from build123d import *

# Parameters (mm, degrees)
SKETCH1_W           = 13
SKETCH1_H           = 12
BOSS_EXTRUDE1_DEPTH = 3
SKETCH2_W           = 13
SKETCH2_H           = 1.9
BOSS_EXTRUDE2_DEPTH = 3
CHAMFER1_SIZE       = 13
CHAMFER1_SIZE_2     = 2
CUT_EXTRUDE1_REACH  = 17.129
CUT_EXTRUDE1_START  = -0.5


with BuildPart() as part:
    # Sketch1 → Boss-Extrude1 (new body)
    with BuildSketch(Plane(origin=(0, 0, 0), x_dir=(1, 0, 0), z_dir=(0, 1, 0))):
        Rectangle(SKETCH1_W, SKETCH1_H)
    extrude(amount=BOSS_EXTRUDE1_DEPTH)

    # Sketch2 → Boss-Extrude2 (add)
    with BuildSketch(Plane.XZ):
        with Locations((0, 5.05)):
            Rectangle(SKETCH2_W, SKETCH2_H)
        with Locations((0, -5.05)):
            Rectangle(SKETCH2_W, SKETCH2_H)
    extrude(amount=BOSS_EXTRUDE2_DEPTH)

    # Chamfer1
    # the kernel refuses this chamfer: 13, 2 mm, written as the material it takes off along each edge
    with BuildSketch(Plane(origin=(6.5, -3, 39.785461495), x_dir=(-0.9999828835142526, -0.005850869894363576, 0), z_dir=(0, 0, -1))) as chamfer1_piece_1:
        Polygon((CHAMFER1_SIZE * 0.999982883514, CHAMFER1_SIZE * 0.00585086989436), (-CHAMFER1_SIZE_2 * 0.00585086989436, CHAMFER1_SIZE_2 * 0.999982883514), (0, 0), align=None)
    extrude(amount=69.470922991, mode=Mode.SUBTRACT)
    with BuildSketch(Plane(origin=(6.5, -3, -39.785461495), x_dir=(-0.9999828835142526, -0.005850869894363576, 0), z_dir=(0, 0, 1))) as chamfer1_piece_2:
        Polygon((CHAMFER1_SIZE * 0.999982883514, -CHAMFER1_SIZE * 0.00585086989436), (-CHAMFER1_SIZE_2 * 0.00585086989436, -CHAMFER1_SIZE_2 * 0.999982883514), (0, 0), align=None)
    extrude(amount=69.470922991, mode=Mode.SUBTRACT)
    with BuildSketch(Plane(origin=(6.5, 3, 39.785461495), x_dir=(0.23997968203750644, -0.9707779108576674, 0), z_dir=(0, 0, -1))) as chamfer1_piece_3:
        Polygon((CHAMFER1_SIZE_2 * 0.970777910858, CHAMFER1_SIZE_2 * 0.239979682038), (-CHAMFER1_SIZE * 0.239979682038, CHAMFER1_SIZE * 0.970777910858), (0, 0), align=None)
    extrude(amount=79.570922991, mode=Mode.SUBTRACT)

    # Sketch5 → Cut-Extrude1 (cut, up to next)
    with BuildSketch(Plane.ZY.offset(6.5).offset(CUT_EXTRUDE1_START), mode=Mode.PRIVATE) as cut_extrude1_sk1:
        with BuildLine():
            Line((-2, 3), (2, 3))
            ThreePointArc((2, 3), (0, 1), (-2, 3))
        make_face()
    cut_extrude1_tool1 = extrude(cut_extrude1_sk1.sketch, amount=-CUT_EXTRUDE1_REACH, mode=Mode.PRIVATE) & part.part
    add(cut_extrude1_tool1.solids().sort_by_distance((-6, 2.151174, 0))[0], mode=Mode.SUBTRACT)


solid = part.part
CAD build for the part. Positions are in the model's coordinates, mm. A direction names the side the tool comes from. Coordinates: 2 decimals unless noted, no trailing zeros. Loops run counter-clockwise (first coordinate to the right, second up) from the corner with the lowest first, then second, coordinate; pieces in that order, holes last. Notation, with made-up numbers: (66, 42) - (121, 42) arc R29 cw to (121, 79) - close; hole circle Ø4 at (4, -31). An arc over 180 degrees is marked (long way). Use one line per item in the form item = value. Start each with the question number.
1) Band-saw the part on D-D (z = 5). Give the cut face in (x, y), and give its area (3 significant figures).
2) Band-saw the part on A-A (x = 4.25). Give the cut face in (y, z).
3) Two-plate mould, pull along Z, no slides. Class faces 4 (the face through (-6, 2, 0)), 5 (the face through (6.5, 0.2, -0.1)), 6 (the face through (0, 0, 0)), 7 (the face through (-2, 0, 6)): +Z half, -Z half, draft (parallel to the pull), parting line (faces both ways), or undercut.
4) Band-saw the part on B-B (z = 0.75). Give the cut face in (x, y).
5) Tool access for faces 1 (the face through (-1, 1, 0)), 2 (the face through (-2, 0, -6)), 3 (the face through (-2, -1, -4.1)): list every direction of +Z, -Z, +X, -X, +Y, -Y with a clear straight run to the whole face (end or side of a thin tool).
6) Band-saw the part on C-C (y = 2.5). Give the cut face in (x, z), and give its area (3 significant figures).
7) Flat gauge pins, fed straight in: pin 1 (1 mm diameter, centred on y = -2, z = 4, fed in from -X); pin 2 (1.5 mm diameter, centred on x = -4, z = 2.5, fed in from -Y). Where does each tip first touch, or does it go through?
8) Drill centre lines: L1, parallel to Z at x = 4.75, y = -0.25; L2, parallel to Y at x = 0, z = 3.75; L3, parallel to X at y = 2.5, z = 1.5. Where is each one in solid material? Low to high. Write a range as from..to.
Check values:
q1.outline = (-6.5, -3) - (6.5, -1) - (6.5, 1) - (-6.5, 3) - close
q1.area = 52.0 mm2
q2.outline = (-1.35, -6) - (1.35, -6) - (1.35, -1.12) arc R2 cw to (1.35, 1.12) - (1.35, 6) - (-1.35, 6) - (-1.35, 4.1) - (0, 4.1) - (0, -4.1) - (-1.35, -4.1) - close
q3.face_4 = undercut
q3.face_5 = draft
q3.face_6 = undercut
q3.face_7 = +Z half
q4.outline = (-6.5, 0) - (6.5, 0) - (6.5, 1) - (5.55, 1.15) - (-6, 1.15) - (-6, 2.92) - (-6.5, 3) - close
q5.face_1 = +X, +Y
q5.face_2 = -Z, +X, -X, +Y, -Y
q5.face_3 = +X, -X, -Y
q6.outline = (-6.5, -6) - (-3.25, -6) - (-3.25, -1.94) - (-6, -1.94) - (-6, 1.94) - (-3.25, 1.94) - (-3.25, 6) - (-6.5, 6) - close
q6.area = 28.3 mm2
q7.pin_1 = -6.5
q7.pin_2 = 0
q8.L1 = -6..-4.1, 4.1..6
q8.L2 = 0..2
q8.L3 = -6.5..-6
